For this review, take the finished solid that the model builds, in its own axes (mm). Face numbers are marked on the shaded views. Round coordinates to 2 decimals unless told otherwise and drop trailing zeros. Loops run counter-clockwise (first coordinate to the right, second up) from the corner with the lowest first, then second, coordinate; pieces in that order, holes last.
1. Consider section B-B on x = 25.5. State the section outline as (y, z) points.
2. Draft analysis for pull direction X (two halves, no side actions). For the marked faces 1, 2 and 3, state which applies: released by +X, released by -X, zero draft, split by the parting line, or undercut.
3. Consider section C-C on z = 7. State the section outline as (x, y) points, then the cut area to 3 significant figures.
4. Consider section D-D on x = 12. State the section outline as (y, z) points, then the cut area to 3 significant figures.
5. Consider section A-A on z = -3. State the section outline as (x, y) points, then the cut area to 3 significant figures.
6. To check wall thickness, follow line 1 along Z through (x, y) = (25.5, 2.6); line 2 along Z through (x, y) = (17, 2.35); line 3 along X through (y, z) = (3.6, -7). State the ranges of each line that lie inside material, in increasing order.
7. Clearance check with flat-ended pins moving along their axes: pin 1 Ø4 at (x, z) = (-20.11, -17.83) entering from -Y; pin 2 Ø2 at (x, y) = (26.5, 3) entering from -Z. State where each tip first meets the part, or that it passes through.
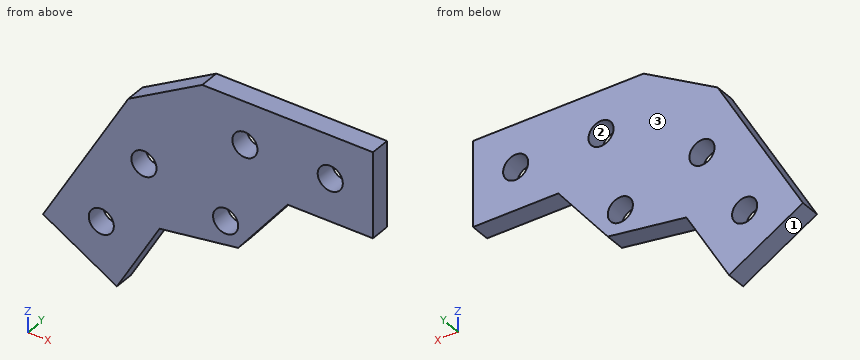
from build123d import *

# Parameters (mm, degrees)
SKETCH1_W           = 34
SKETCH1_H           = 17
SKETCH1_R           = 2.5
BOSS_EXTRUDE1_DEPTH = 4
BOSS_EXTRUDE2_DEPTH = 4
SKETCH13_R          = 2.5
BOSS_EXTRUDE3_DEPTH = 4


with BuildPart() as part:
    # sketch1 → Boss-Extrude1 (new body)
    with BuildSketch(Plane(origin=(0, 0, 0), x_dir=(1, 0, 0), z_dir=(0, 1, 0))):
        with Locations((17, -8.5)):
            Rectangle(SKETCH1_W, SKETCH1_H)
        with Locations((8.5, -8.5)):
            Circle(SKETCH1_R, mode=Mode.SUBTRACT)
        with Locations((25.5, -8.5)):
            Circle(SKETCH1_R, mode=Mode.SUBTRACT)
    extrude(amount=BOSS_EXTRUDE1_DEPTH)


with BuildPart() as body_2:
    # Mirror6: mirrored copy
    add(part.part.mirror(Plane(origin=(0, 0, 0), x_dir=(-0.5, 0, 0.866025404), z_dir=(-0.866025404, 0, -0.5))))


with BuildPart() as part_1:
    add(part.part)

    add(body_2.part)  # Boss-Extrude2 merges body 2
    # Sketch11 → Boss-Extrude2 (add)
    with BuildSketch(Plane(origin=(0, 0, 0), x_dir=(1, 0, 0), z_dir=(0, 1, 0))):
        Polygon((-14.722431864, -8.5), (0, -17), (0, 0), align=None)
    extrude(amount=BOSS_EXTRUDE2_DEPTH)

    # Sketch13 → Boss-Extrude3 (add)
    with BuildSketch(Plane(origin=(0, 0, 0), x_dir=(1, 0, 0), z_dir=(0, 1, 0))):
        Polygon((7.152847248, 12.389094852), (-8.5, 14.722431864), (0, 0), (17, 0), align=None)
        with Locations((4.652847248, 8.058967833)):
            Circle(SKETCH13_R, mode=Mode.SUBTRACT)
    extrude(amount=BOSS_EXTRUDE3_DEPTH)


solid = part_1.part
Resolved:
1. outline: (0, 0) - (4, 0) - (4, 6) - (0, 6) - close; (0, 11) - (4, 11) - (4, 17) - (0, 17) - close
2. face 1: released by -X
2. face 2: undercut
2. face 3: zero draft
3. outline: (-15.59, 0) - (6.5, 0) - (6.5, 4) - (-15.59, 4) - close; (10.5, 0) - (23.5, 0) - (23.5, 4) - (10.5, 4) - close; (27.5, 0) - (34, 0) - (34, 4) - (27.5, 4) - close
3. area: 166 mm2
4. outline: (0, -6.29) - (4, -6.29) - (4, 17) - (0, 17) - close
4. area: 93.2 mm2
5. outline: (-21.36, 0) - (-14.11, 0) - (-14.11, 4) - (-21.36, 4) - close; (-9.11, 0) - (14.62, 0) - (14.62, 4) - (-9.11, 4) - close
5. area: 124 mm2
6. line 1: z = 0 to 6, 11 to 17
6. line 2: z = 0 to 17
6. line 3: x = -23.67 to 2.39, 6.92 to 11.44
7. pin 1: passes through
7. pin 2: stops at z = 0
